Source: CAD feature listing. Evaluate the final solid. Frame: model axes, mm. A direction names the side the tool comes from. Round coordinates to 2 decimals unless told otherwise and drop trailing zeros. Order: outer loops, then holes, each group sorted by start corner. A loop starts at its lowest first (then second) coordinate and runs counter-clockwise, first axis right, second up. Notation, with made-up numbers: M 23,-29.5 L 29,-29.5 A31 cw 29,4.5 Z; hole C 25,89.5 d5. An arc over 180 degrees is marked long. Answer as CSV lines item,"result". Start each with the question number.
Item 1: Section query A-A on z = 0. Return the cut outline in (x, y), plus the area to 3 significant figures.
Item 2: Set-up query: faces 1 (the face through (-17.59, 5.86, 13.48)), 2 (the face through (-3.964, 12.482, 17.853)). Return all of +Z, -Z, +X, -X, +Y, -Y with unobstructed straight access to the full face (end or side cutting, diameter ignored); none if empty.
Item 3: Section query B-B on x = 0. Return the cut outline in (y, z).
Item 4: Line query: line 1 (X direction, y = 7, z = 0.5); line 2 (X direction, y = 11.3, z = 0). Output: solid intervals per line, ascending. Write a range as [from, to].
Item 5: Pull-direction query (Z, two-part tool) for faces 3 (the face through (21.405, 5.801, -6.741)), 4 (the face through (-3.9, 12.47, 17.58)); classes: +Z half, -Z half, draft (parallel to the pull), parting line (faces both ways), or undercut.
Item 6: First-contact query: P1, Ø1.5, axis at y = 12.5, z = -15, coming from the -X side; P2, Ø13, axis at x = -9, z = -4, coming from the +Y side; P3, Ø6, axis at x = -16.5, y = 7, coming from the +Z side; P4, Ø3, axis at x = 5.5, y = 11.5, coming from the +Z side. Flat tips, straight axial feed; report the tip coordinate or a pass-through.
from build123d import *


with BuildPart() as part:
    # Sketch1 → Revolve1 (revolve)
    with BuildSketch(Plane(origin=(0, 0, 0), x_dir=(-1, 0, 0), z_dir=(0, 0, -1))):
        with BuildLine():
            Line((-21.5265, 8.1026), (-18.0086, 10.133660512))
            Line((-18.0086, 10.133660512), (-18.0086, 14.732))
            Line((-18.0086, 14.732), (-18.288, 14.732))
            Line((-18.288, 14.732), (-18.288, 10.294972177))
            Line((-18.288, 10.294972177), (-21.601365004, 8.382))
            Line((-21.601365004, 8.382), (-21.9075, 8.382))
            ThreePointArc((-21.9075, 8.382), (-22.284670757, 8.225770757), (-22.4409, 7.8486))
            Line((-22.4409, 7.8486), (-22.4409, 3.81))
            Line((-22.4409, 3.81), (-22.1615, 3.81))
            Line((-22.1615, 3.81), (-22.1615, 7.8486))
            ThreePointArc((-22.1615, 7.8486), (-22.087105122, 8.028205122), (-21.9075, 8.1026))
            Line((-21.9075, 8.1026), (-21.5265, 8.1026))
        make_face()
    revolve(axis=Axis((0, 3.81, 0), (0, 1, 0)))


solid = part.part
Results:
1,outline,"M -22.44,3.81 L -22.16,3.81 L -22.16,7.85 A0.25 cw -21.91,8.1 L -21.53,8.1 L -18.01,10.13 L -18.01,14.73 L -18.29,14.73 L -18.29,10.29 L -21.6,8.38 L -21.91,8.38 A0.53 ccw -22.44,7.85 Z; M 18.01,10.13 L 21.53,8.1 L 21.91,8.1 A0.25 cw 22.16,7.85 L 22.16,3.81 L 22.44,3.81 L 22.44,7.85 A0.53 ccw 21.91,8.38 L 21.6,8.38 L 18.29,10.29 L 18.29,14.73 L 18.01,14.73 Z"
1,area,"7.52 mm^2"
2,face 1,"-Y"
2,face 2,"+Y"
3,outline,"M 3.81,-22.44 L 7.85,-22.44 A0.53 ccw 8.38,-21.91 L 8.38,-21.6 L 10.29,-18.29 L 14.73,-18.29 L 14.73,-18.01 L 10.13,-18.01 L 8.1,-21.53 L 8.1,-21.91 A0.25 cw 7.85,-22.16 L 3.81,-22.16 Z; M 3.81,22.16 L 7.85,22.16 A0.25 cw 8.1,21.91 L 8.1,21.53 L 10.13,18.01 L 14.73,18.01 L 14.73,18.29 L 10.29,18.29 L 8.38,21.6 L 8.38,21.91 A0.53 ccw 7.85,22.44 L 3.81,22.44 Z"
4,line 1,"[-22.44, -22.16], [22.16, 22.44]"
4,line 2,"[-18.29, -18.01], [18.01, 18.29]"
5,face 3,"parting line"
5,face 4,"undercut"
6,P1,"x = -11.46"
6,P2,"through"
6,P3,"z = 17.93"
6,P4,"z = 18.01"
